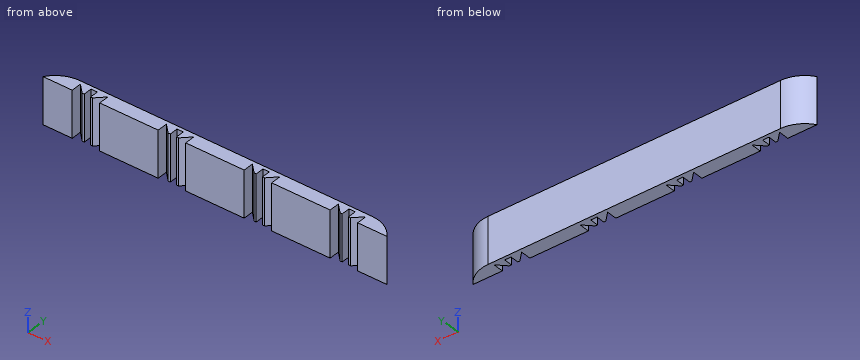
```python
from build123d import *

# Parameters (mm, degrees)
SKETCH1_W           = 254
SKETCH1_H           = 34.29
BOSS_EXTRUDE1_DEPTH = 10.16
FILLET1_R           = 22.86
CUT_EXTRUDE2_DEPTH  = 50.8
LPATTERN1_COUNT     = 4
LPATTERN1_PITCH     = 63.5


with BuildPart() as part:
    # Sketch1 → Boss-Extrude1 (new body)
    with BuildSketch(Plane(origin=(0, 0, 0), x_dir=(1, 0, 0), z_dir=(0, 1, 0))):
        Rectangle(SKETCH1_W, SKETCH1_H)
    extrude(amount=BOSS_EXTRUDE1_DEPTH)

    # Fillet1
    # the kernel refuses this fillet: 22.86 mm, written as the material it takes off along each edge
    with BuildSketch(Plane(origin=(-127, 10.16, 64.664048812), x_dir=(0, -1, 0), z_dir=(0, 0, -1)), Plane(origin=(127, 10.16, -64.664048812), x_dir=(0, -1, 0), z_dir=(0, 0, 1))) as fillet1_piece_1:
        with BuildLine():
            CenterArc((22.86, -19.007619525), FILLET1_R, 123.748988596, 56.251011404)
            Line((0, -19.007619525), (-0.4572, -19.007619525))
            Line((-0.4572, -19.007619525), (-0.4572, 0))
            Line((-0.4572, 0), (0, 0.4572))
            ThreePointArc((0, 0.4572), (5.08, 0.4572), (9.906, 0.38015239))
            Line((9.906, 0.38015239), (10.16, 0))
        make_face()
    extrude(amount=129.328097624, mode=Mode.SUBTRACT)

    # Sketch2 → Cut-Extrude2 (cut)
    with BuildSketch(Plane.XY.offset(17.145)):
        Polygon((-85.09, 0), (-85.09, 7.62), (-91.35478418, 1.35521582), (-92.92396906, 1.35521582), (-92.92396906, 7.62), (-97.57603094, 7.62), (-97.57603094, 1.35521582), (-99.14521582, 1.35521582), (-105.41, 7.62), (-105.41, 0), align=None)
    cut_extrude2 = extrude(amount=-CUT_EXTRUDE2_DEPTH, mode=Mode.SUBTRACT)

    # LPattern1: Cut-Extrude2 ×4
    with Locations(*[(i * LPATTERN1_PITCH, 0, 0) for i in range(1, LPATTERN1_COUNT)]):
        add(cut_extrude2, mode=Mode.SUBTRACT)


solid = part.part
```
Could you check a few things on this model? Use its own coordinates, in mm. Give positions to 0.01 mm unless a question says otherwise; leave off trailing zeros. Write each loop counter-clockwise with the first axis right and the second up, starting at its lowest first coordinate (ties: lowest second). Pieces come first, ordered by that corner, then holes. Notation, with made-up numbers: (-8.75, -11) -> (12.25, -11) arc R24 ccw to (12.25, 24) -> close; hole circle Ø4 at (56.5, 67.5). An arc over 180 degrees is marked (long way). Write each question's results on one line, items separated by ' | '.
1. I want a section at A-A, the plane y = 4.5. Count the separate pieces of the cut face and the enclosed holes in it, then the cut area to 3 significant figures.
Check sheet entries:
separate pieces: 13 | enclosed holes: 0 | area: 6,940 mm²
2. I want a section at B-B, the plane x = 88. Write out the boundary of the cut face in (y, z) (3 decimals).
Check sheet entries:
outline: (4.71, -17.145) -> (10.16, -17.145) -> (10.16, 17.145) -> (4.71, 17.145) -> close
3. I need wall thicknesses on L1, parallel to X at y = 1, z = -4; L2, parallel to Y at x = 35, z = 16.5; L3, parallel to Y at x = 95.5, z = -13.5. Which ranges of each line are inside material? Lowest first, please.
Check sheet entries:
L1: x = -126.29 to -105.41, -85.09 to -41.91, -21.59 to 21.59, 41.91 to 85.09, 105.41 to 126.29 | L2: y = 1.36 to 10.16 | L3: y = 7.62 to 10.16
4. Will these pins go through, and if not, where does the flat tip stop? pin 1 Ø1.3 at (x, z) = (35, -4.5) entering from -Y; pin 2 Ø2.5 at (y, z) = (5, -5) entering from +X; pin 3 Ø1.9 at (y, z) = (5.5, 4.5) entering from +X; pin 4 Ø1.5 at (x, z) = (-5.5, -2.5) entering from -Y.
Check sheet entries:
pin 1: stops at y = 1.36 | pin 2: stops at x = 123.87 | pin 3: stops at x = 122.99 | pin 4: stops at y = 0
